Here's how the part is built. I have some questions about the finished solid (model axes, mm). Round coordinates to 2 decimals unless told otherwise and drop trailing zeros. Order: outer loops, then holes, each group sorted by start corner. A loop starts at its lowest first (then second) coordinate and runs counter-clockwise, first axis right, second up. Notation, with made-up numbers: (78, -9) - (130, -9) arc R7 cw to (130, -1) - close; hole circle Ø3 at (44.5, -6.5). An arc over 180 degrees is marked (long way). Answer as a JSON object with one key per item and string values.
```python
from build123d import *

# Parameters (mm, degrees)
SKETCH1_W           = 40
SKETCH1_H           = 262
SKETCH1_R           = 1.25
BOSS_EXTRUDE1_DEPTH = 2.5
SKETCH2_R           = 5
SKETCH2_R_2         = 1.6
SKETCH2_R_3         = 2
SKETCH2_R_4         = 3.5
CUT_EXTRUDE1_DEPTH  = 3.5
SKETCH3_W           = 20.5
SKETCH3_H           = 17.5
CUT_EXTRUDE2_DEPTH  = 3.5


with BuildPart() as part:
    # Sketch1 → Boss-Extrude1 (new body)
    with BuildSketch(Plane.XY):
        with Locations((20, 131)):
            Rectangle(SKETCH1_W, SKETCH1_H)
        with Locations((12.65, 258.7)):
            Circle(SKETCH1_R, mode=Mode.SUBTRACT)
        with Locations((12.65, 3.3)):
            Circle(SKETCH1_R, mode=Mode.SUBTRACT)
    extrude(amount=BOSS_EXTRUDE1_DEPTH)

    # Sketch2 → Cut-Extrude1 (cut, through all)
    with BuildSketch(Plane.XY.offset(2.5)):
        with Locations((20, 55.004773675)):
            Circle(SKETCH2_R)
        with Locations((20, 64.504773675)):
            Circle(SKETCH2_R_2)
        with Locations((5, 96)):
            Circle(SKETCH2_R_3)
        with Locations((26.5, 90)):
            Circle(SKETCH2_R_3)
        with Locations((36.5, 177)):
            Circle(SKETCH2_R_3)
        with Locations((6, 183.25)):
            Circle(SKETCH2_R_3)
        with Locations((7.75, 202)):
            Circle(SKETCH2_R_4)
        with BuildLine():
            Line((6.080589093, 233.49778539), (4.080589089, 233.49778539))
            Line((4.080589089, 233.49778539), (4.080589089, 236.49778539))
            Line((4.080589089, 236.49778539), (6.080589093, 236.49778539))
            ThreePointArc((6.080589093, 236.49778539), (34, 234.99778539), (6.080589093, 233.49778539))
        make_face()
    extrude(amount=-CUT_EXTRUDE1_DEPTH, mode=Mode.SUBTRACT)

    # Sketch3 → Cut-Extrude2 (cut, through all)
    with BuildSketch(Plane.XY.offset(2.5)):
        with Locations((29.75, 8.75)):
            Rectangle(SKETCH3_W, SKETCH3_H)
    extrude(amount=-CUT_EXTRUDE2_DEPTH, mode=Mode.SUBTRACT)


solid = part.part
```
1. Imagine slicing it at A-A (y = 227.5). List the corners of the cut face in (x, z) for me.
Responses:
{"outline": "(0, 0) - (8.18, 0) - (8.18, 2.5) - (0, 2.5) - close; (31.82, 0) - (40, 0) - (40, 2.5) - (31.82, 2.5) - close"}
2. Imagine slicing it at B-B (z = 2.1). Give the number of separate pieces and of enclosed holes in the cut face, plus the area to 3 significant figures.
Responses:
{"separate pieces": "1", "enclosed holes": "10", "area": "9,310 mm2"}
3. For P1, Ø0.8, axis at y = 11.5, z = 1, coming from the +X side; P2, Ø4, axis at x = 12.65, y = 258.7, coming from the -Z side, each with a flat end and sliding along its axis, tell me the tip position at first contact or that it passes through.
Responses:
{"P1": "x = 19.5", "P2": "z = 0"}
4. Thinking about a two-plate mould opening in X: for faces 1 (the face through (6.991, 198.583, 1.268)), 2 (the face through (20, 133, 2.5)), which applies, pulls with the +X half, pulls with the -X half, needs draft (parallel to the pull), parting line crosses it, or undercut?
Responses:
{"face 1": "undercut", "face 2": "needs draft"}
5. If I drill on L1, parallel to Y at x = 20, z = 1.4; L2, parallel to Y at x = 36.5, z = 0.65; L3, parallel to Y at x = 5, z = 1.95, over which ranges is the centre line in solid material (lowest first)? Write a range as [from, to].
Responses:
{"L1": "[17.5, 50], [60, 62.9], [66.1, 221], [249, 262]", "L2": "[17.5, 175], [179, 262]", "L3": "[0, 94], [98, 181.52], [184.98, 199.83], [204.17, 233.5], [236.5, 262]"}
